```python
from build123d import *

# Parameters (mm, degrees)
SKETCH_1_R             = 1.75
SKETCH_1_R_2           = 4
SKETCH_1_R_3           = 1.55
SKETCH_1_R_4           = 5
SKETCH_1_R_5           = 2.55
EXTRUDE_1_DEPTH        = 3
FILLET_1_R             = 10
SKETCH_2_R             = 1.75
CUT_EXTRUDE_1_DEPTH    = 3
CUT_EXTRUDE_2_DEPTH    = 10
FILLET_2_R             = 2
FILLET_2_OF_MIRROR_2_R = 2
SKETCH_5_R             = 12.5
CUT_EXTRUDE_3_DEPTH    = 10
EXTRUDE_2_DEPTH        = 3
FILLET_3_R             = 2
FILLET_4_R             = 2


with BuildPart() as part:
    # 草图1 → 凸台-拉伸1 (new body)
    # profile 1 of 3: a face of its own
    with BuildSketch(Plane.XY):
        with BuildLine():
            ThreePointArc((-31.074028853, 87.25), (-35.139866152, 83.250541855), (-39.071861578, 87.38165676))
            Line((-39.071861578, 87.38165676), (-40.590218292, 41.27588782))
            ThreePointArc((-40.590218292, 41.27588782), (-41.439715326, 35.904074252), (-43.581025503, 30.904792609))
            Line((-43.581025503, 30.904792609), (-54.317561995, 12.521638043))
            ThreePointArc((-54.317561995, 12.521638043), (-48.693824279, 14.826375968), (-45, 10))
            ThreePointArc((-45, 10), (-46.464466094, 6.464466094), (-50, 5))
            Line((-50, 5), (0, 5))
            Line((0, 5), (0, 82))
            Line((0, 82), (-34.039489079, 91.113900549))
            ThreePointArc((-34.039489079, 91.113900549), (-31.900847556, 89.685348117), (-31.074028853, 87.25))
        make_face()
        with Locations((-12.07, 35)):
            Circle(SKETCH_1_R, mode=Mode.SUBTRACT)
        with Locations((-12.07, 61)):
            Circle(SKETCH_1_R, mode=Mode.SUBTRACT)
    # profile 2 of 3: a face of its own
    with BuildSketch(Plane.XY):
        with Locations((-35.074028853, 87.25)):
            Circle(SKETCH_1_R_2)
        with Locations((-35.074028853, 87.25)):
            Circle(SKETCH_1_R_3, mode=Mode.SUBTRACT)
    # profile 3 of 3: a face of its own
    with BuildSketch(Plane.XY):
        with Locations((-50, 10)):
            Circle(SKETCH_1_R_4)
        with Locations((-50, 10)):
            Circle(SKETCH_1_R_5, mode=Mode.SUBTRACT)
    extrude_1 = extrude(amount=EXTRUDE_1_DEPTH)

    # 镜向1: 凸台-拉伸1 across plane
    add(extrude_1.mirror(Plane(origin=(0, 0, 3), x_dir=(0, 0, 1), z_dir=(-1, 0, 0))))

    # 圆角1
    fillet_1_edges = [part.edges().sort_by_distance(p)[0] for p in [
        (0, 82, 1.5),
    ]]
    fillet(fillet_1_edges, radius=FILLET_1_R)

    # 草图2 → 切除-拉伸1 (cut)
    with BuildSketch(Plane.XY.offset(3)):
        with Locations((0, 10)):
            Circle(SKETCH_2_R)
    extrude(amount=-CUT_EXTRUDE_1_DEPTH, mode=Mode.SUBTRACT)

    # 草图4 → 切除-拉伸2 (cut)
    with BuildSketch(Plane.XY.offset(3)):
        with BuildLine():
            ThreePointArc((-10.354163178, 65.111145633), (-7.386964112, 66.58582151), (-4.21701247, 67.550365875))
            Line((-4.21701247, 67.550365875), (-4.21701247, 76.60212181))
            Line((-4.21701247, 76.60212181), (-25.392834673, 82.271840799))
            Line((-25.392834673, 82.271840799), (-10.354163178, 65.111145633))
        make_face()
        with BuildLine():
            ThreePointArc((-16.581442579, 36.817166638), (-19.997686263, 48.304210684), (-16.233615619, 59.682025678))
            Line((-16.233615619, 59.682025678), (-31.409439241, 76.999225749))
            Line((-31.409439241, 76.999225749), (-32.594552841, 41.0125743))
            ThreePointArc((-32.594552841, 41.0125743), (-33.411565317, 34.978483904), (-35.430174477, 29.233662466))
            Line((-35.430174477, 29.233662466), (-38.728362293, 22.219935083))
            Line((-38.728362293, 22.219935083), (-16.581442579, 36.817166638))
        make_face()
        with BuildLine():
            Line((-4, 13), (-4, 28.404082058))
            ThreePointArc((-4, 28.404082058), (-7.476808875, 29.45013938), (-10.707211367, 31.107527572))
            Line((-10.707211367, 31.107527572), (-12.178851974, 30.137556172))
            Line((-12.178851974, 30.137556172), (-34.325771688, 15.540324618))
            Line((-34.325771688, 15.540324618), (-38.179952199, 13))
            Line((-38.179952199, 13), (-4, 13))
        make_face()
    cut_extrude_2 = extrude(amount=-CUT_EXTRUDE_2_DEPTH, mode=Mode.SUBTRACT)

    # 圆角2
    fillet_2_edges = [part.edges().sort_by_distance(p)[0] for p in [
        (-31.409439241, 76.999225749, 1.5),
        (-16.233615619, 59.682025678, 1.5),
        (-16.581442579, 36.817166638, 1.5),
        (-38.728362293, 22.219935083, 1.5),
        (-10.707211367, 31.107527572, 1.5),
        (-4, 28.404082058, 1.5),
        (-4, 13, 1.5),
        (-38.179952199, 13, 1.5),
        (-4.21701247, 67.550365875, 1.5),
        (-10.354163178, 65.111145633, 1.5),
        (-25.392834673, 82.271840799, 1.5),
        (-4.21701247, 76.60212181, 1.5),
    ]]
    fillet(fillet_2_edges, radius=FILLET_2_R)

    # 镜向2: 切除-拉伸2 across plane
    add(cut_extrude_2.mirror(Plane(origin=(0, 0, 0), x_dir=(0, 0, 1), z_dir=(1, 0, 0))), mode=Mode.SUBTRACT)

    # 圆角2 of 镜向2
    fillet_2_of_mirror_2_edges = [part.edges().sort_by_distance(p)[0] for p in [
        (31.409439241, 76.999225749, 1.5),
        (16.233615619, 59.682025678, 1.5),
        (16.581442579, 36.817166638, 1.5),
        (38.728362293, 22.219935083, 1.5),
        (10.707211367, 31.107527572, 1.5),
        (4, 28.404082058, 1.5),
        (4, 13, 1.5),
        (38.179952199, 13, 1.5),
        (4.21701247, 67.550365875, 1.5),
        (10.354163178, 65.111145633, 1.5),
        (25.392834673, 82.271840799, 1.5),
        (4.21701247, 76.60212181, 1.5),
    ]]
    fillet(fillet_2_of_mirror_2_edges, radius=FILLET_2_OF_MIRROR_2_R)

    # 草图5 → 切除-拉伸3 (cut)
    with BuildSketch(Plane.XY.offset(3)):
        with Locations((0, 48)):
            Circle(SKETCH_5_R)
    extrude(amount=-CUT_EXTRUDE_3_DEPTH, mode=Mode.SUBTRACT)

    # 草图6 → 凸台-拉伸2 (add)
    with BuildSketch(Plane.XY.offset(3)):
        with BuildLine():
            Line((-32.364442706, 48), (-20, 48))
            ThreePointArc((-20, 48), (-19.89872306, 50.01017924), (-19.595917942, 52))
            Line((-19.595917942, 52), (-32.232714574, 52))
            Line((-32.232714574, 52), (-32.364442706, 48))
        make_face()
        with BuildLine():
            ThreePointArc((-19.595917942, 44), (-19.89872306, 45.98982076), (-20, 48))
            Line((-20, 48), (-32.364442706, 48))
            Line((-32.364442706, 48), (-32.496170839, 44))
            Line((-32.496170839, 44), (-19.595917942, 44))
        make_face()
    extrude_2 = extrude(amount=-EXTRUDE_2_DEPTH)

    # 镜向3: 凸台-拉伸2 across plane
    add(extrude_2.mirror(Plane(origin=(0, 0, 0), x_dir=(0, 0, 1), z_dir=(1, 0, 0))))

    # 圆角3
    fillet_3_edges = [part.edges().sort_by_distance(p)[0] for p in [
        (-19.595917942, 52, 1.5),
        (-19.595917942, 44, 1.5),
        (-32.496170839, 44, 1.5),
        (-32.232714574, 52, 1.5),
    ]]
    fillet(fillet_3_edges, radius=FILLET_3_R)

    # 圆角4
    fillet_4_edges = [part.edges().sort_by_distance(p)[0] for p in [
        (19.595917942, 44, 1.5),
        (19.595917942, 52, 1.5),
        (32.232714574, 52, 1.5),
        (32.496170839, 44, 1.5),
    ]]
    fillet(fillet_4_edges, radius=FILLET_4_R)


solid = part.part
```
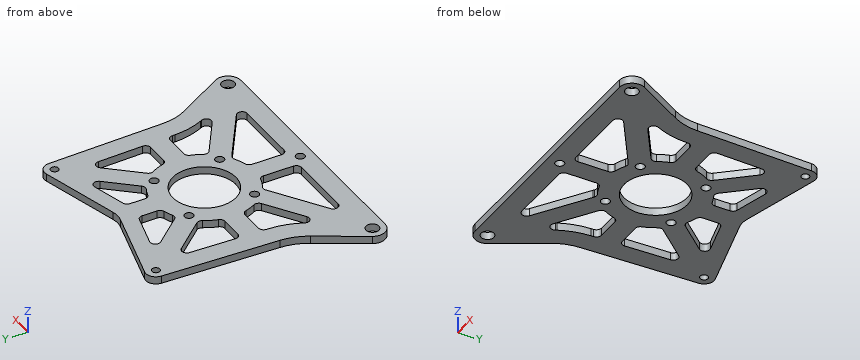
Part model, mm, in its own coordinate system. Coordinates: 2 decimals unless noted, no trailing zeros. Order: outer loops, then holes, each group sorted by start corner. A loop starts at its lowest first (then second) coordinate and runs counter-clockwise, first axis right, second up. Notation, with made-up numbers: (-38.5, -25.5) - (-28.5, -25.5) arc R20 cw to (-28.5, -1.5) - close; hole circle Ø5 at (55, 49). An arc over 180 degrees is marked (long way). Return JSON: item names as keys, results as strings. Group by question number.
Item 1: Cut at B-B (y = 10). List the corners of the cut face in (x, z), plus the area to 3 significant figures.
Item 2: Pin check, flat tips, straight feed: pin 1 (2 mm diameter, centred on x = -12.07, y = 35, fed in from +Z); pin 2 (1.5 mm diameter, centred on x = 13.5, z = 1.5, fed in from +Y); pin 3 (0.9 mm diameter, centred on y = 73.5, z = 2, fed in from -X); pin 4 (0.9 mm diameter, centred on y = 73, z = 1.5, fed in from +X). Stop position of each tip, or through.
Item 3: Cut at C-C (x = -23). List the corners of the cut face in (y, z), plus the area to 3 significant figures.
Item 4: Cut at D-D (y = 48). List the corners of the cut face in (x, z), plus the area to 3 significant figures.
Item 5: Drill centre lines: probe 1 along Y at (x, z) = (7, 1.1) (3 decimals); probe 2 along Y at (x, z) = (-26, 0.3); probe 3 along Y at (x, z) = (18.5, 2.5). Where is each one in solid material? Low to high. Write a range as from..to.
Item 6: Cut at A-A (x = 0). List the corners of the cut face in (y, z).
Check values:
{
 "1": {"outline": "(-55, 0) - (-52.55, 0) - (-52.55, 3) - (-55, 3) - close; (-47.45, 0) - (-1.75, 0) - (-1.75, 3) - (-47.45, 3) - close; (1.75, 0) - (47.45, 0) - (47.45, 3) - (1.75, 3) - close; (52.55, 0) - (55, 0) - (55, 3) - (52.55, 3) - close", "area": "289 mm2"},
 "2": {"pin 1": "passes through", "pin 2": "stops at y = 85.82", "pin 3": "stops at x = -39.54", "pin 4": "stops at x = 39.56"},
 "3": {"outline": "(5, 0) - (13, 0) - (13, 3) - (5, 3) - close; (23.01, 0) - (32.59, 0) - (32.59, 3) - (23.01, 3) - close; (44, 0) - (52, 0) - (52, 3) - (44, 3) - close; (67.4, 0) - (88.16, 0) - (88.16, 3) - (67.4, 3) - close", "area": "139 mm2"},
 "4": {"outline": "(-40.37, 0) - (-12.5, 0) - (-12.5, 3) - (-40.37, 3) - close; (12.5, 0) - (40.37, 0) - (40.37, 3) - (12.5, 3) - close", "area": "167 mm2"},
 "5": {"probe 1": "y = 5..13, 29.265..37.644, 58.356..66.735, 77.347..83.874", "probe 2": "y = 5..13, 21.03..30.61, 44..52, 70.83..88.96", "probe 3": "y = 5..13, 25.97..35.55, 40.4..55.6, 62.27..74.41, 80.43..86.95"},
 "6": {"outline": "(5, 0) - (8.25, 0) - (8.25, 3) - (5, 3) - close; (11.75, 0) - (35.5, 0) - (35.5, 3) - (11.75, 3) - close; (60.5, 0) - (82.35, 0) - (82.35, 3) - (60.5, 3) - close"}
}
